Geometry check sheet. Reference: the model listing, model coordinates, mm. Face numbers are marked on the shaded views. A direction names the side the tool comes from. Give positions to 0.01 mm unless a question says otherwise; leave off trailing zeros. Write each loop counter-clockwise with the first axis right and the second up, starting at its lowest first coordinate (ties: lowest second). Pieces come first, ordered by that corner, then holes. Notation, with made-up numbers: M 70,87.5 L 105,87.5 A4 cw 105,92.5 Z; hole C -8.5,31.5 d9. An arc over 180 degrees is marked long. Write each question's results on one line, items separated by ' | '.
```python
from build123d import *

# Parameters (mm, degrees)
SKETCH1_W           = 50
SKETCH1_H           = 50
BOSS_EXTRUDE1_DEPTH = 50
SKETCH3_R           = 18
BOSS_EXTRUDE2_DEPTH = 40
SKETCH4_R           = 18
BOSS_EXTRUDE3_DEPTH = 40
FILLET1_R           = 20


with BuildPart() as part:
    # Sketch1 → Boss-Extrude1 (new body)
    with BuildSketch(Plane(origin=(0, 0, 0), x_dir=(1, 0, 0), z_dir=(0, 1, 0))):
        Rectangle(SKETCH1_W, SKETCH1_H)
    extrude(amount=BOSS_EXTRUDE1_DEPTH)

    # Sketch3 → Boss-Extrude2 (add)
    with BuildSketch(Plane.XY.offset(25)):
        with Locations((0, 25)):
            Circle(SKETCH3_R)
    extrude(amount=BOSS_EXTRUDE2_DEPTH)

    # Sketch4 → Boss-Extrude3 (add)
    with BuildSketch(Plane.XZ):
        with Locations(Location((0, 0, 0), (0, 0, 270))):
            Circle(SKETCH4_R)
    extrude(amount=BOSS_EXTRUDE3_DEPTH)

    # Fillet1
    fillet1_edges = [part.edges().sort_by_distance(p)[0] for p in [
        (25, 50, 0),
        (0, 50, -25),
        (-25, 50, 0),
        (-25, 25, -25),
        (25, 25, -25),
    ]]
    fillet(fillet1_edges, radius=FILLET1_R)


solid = part.part
```
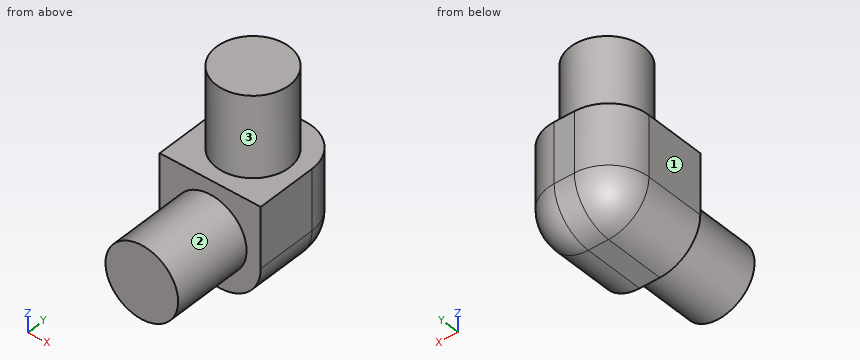
Q1. Section check D-D (x = 11). Enter the section's corners in (y, z), then the cut area to 3 significant figures.
Answer key:
outline: M -40,-14.25 L 0,-14.25 L 0,-24.08 L 30,-24.08 A19.08 ccw 49.08,-5 L 49.08,25 L 39.25,25 L 39.25,65 L 10.75,65 L 10.75,25 L 0,25 L 0,14.25 L -40,14.25 Z | area: 4,610 mm2
Q2. Material ranges on probe 1 along Z at (x, y) = (-1.5, 7); probe 2 along Y at (x, z) = (-11, 4); probe 3 along Z at (x, y) = (8.5, 18.5), recorded low to high. Write a range as [from, to].
Answer key:
probe 1: z = [-25, 25] | probe 2: y = [-40, 49.08] | probe 3: z = [-24.69, 65]
Q3. Section check C-C (y = 25). Enter the section's corners in (x, z).
Answer key:
outline: M -25,-5 A20 ccw -5,-25 L 5,-25 A20 ccw 25,-5 L 25,25 L 18,25 L 18,65 L -18,65 L -18,25 L -25,25 Z
Q4. Section check A-A (x = 0). Enter the section's corners in (y, z).
Answer key:
outline: M -40,-18 L 0,-18 L 0,-25 L 30,-25 A20 ccw 50,-5 L 50,25 L 43,25 L 43,65 L 7,65 L 7,25 L 0,25 L 0,18 L -40,18 Z
Q5. Access from +Z, -Z, +X, -X, +Y, -Y to the whole of each face (thin tool, end or side, straight path). Record for the marked faces 1, 2 and 3.
Answer key:
face 1: +Z, -Z, -X, +Y, -Y | face 2: -Y | face 3: +Z
Q6. Depth check by flat-ended pin: P1, Ø1.5, axis at x = -19.5, z = 15, coming from the -Y side; P2, Ø10, axis at y = 35, z = 15.5, coming from the +X side; P3, Ø5, axis at x = -18, y = 38.5, coming from the +Z side; P4, Ø8, axis at x = 14, z = 31.5, coming from the +Y side. Enter the tip coordinate at first touch or a pass-through.
Answer key:
P1: stops at y = 0 | P2: stops at x = 25 | P3: stops at z = 25 | P4: stops at y = 39.97
Q7. Section check B-B (z = 0). Enter the section's corners in (x, y), then the cut area to 3 significant figures.
Answer key:
outline: M -25,0 L -18,0 L -18,-40 L 18,-40 L 18,0 L 25,0 L 25,30 A20 ccw 5,50 L -5,50 A20 ccw -25,30 Z | area: 3,770 mm2
